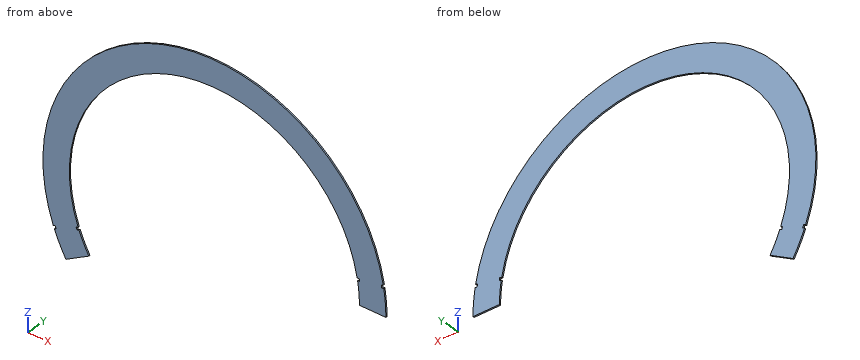
from build123d import *

# Parameters (mm, degrees)
BOSS_EXTRUDE1_DEPTH = 0.7
CUT_EXTRUDE1_DEPTH  = 120.107123213
BOSS_EXTRUDE2_DEPTH = 0.7


with BuildPart() as part:
    # Sketch3 → Boss-Extrude1 (new body)
    with BuildSketch(Plane(origin=(0, 0, 0), x_dir=(1, 0, 0), z_dir=(0, 1, 0))):
        with BuildLine():
            Line((-61.678329258, 35.61), (-72.936659507, 42.11))
            ThreePointArc((-72.936659507, 42.11), (-21.797739979, -81.35027309), (84.22, 0))
            Line((84.22, 0), (71.22, 0))
            ThreePointArc((71.22, 0), (-18.433092392, -68.793237348), (-61.678329258, 35.61))
        make_face()
    extrude(amount=BOSS_EXTRUDE1_DEPTH)

    # Sketch5 → Cut-Extrude1 (cut, through all)
    with BuildSketch(Plane(origin=(0, 0, 0), x_dir=(1, 0, 0), z_dir=(0, 1, 0))):
        Polygon((-66.489597975, 25.522965367), (-80.493304373, 30.89848461), (-81.020297764, 29.488976758), (-66.924908452, 24.358674608), align=None)
    cut_extrude1 = extrude(amount=CUT_EXTRUDE1_DEPTH, mode=Mode.SUBTRACT)


with BuildPart() as cut_extrude1_piece_1:
    # of the separate pieces the step leaves, piece 1, a body of its own (cut_extrude1_pieces)
    add(part.part.solids().sort_by_distance((84.22, 0, 0))[0])



with BuildPart() as cut_extrude1_piece_2:
    # of the separate pieces the step leaves, piece 2, a body of its own (cut_extrude1_pieces)
    add(part.part.solids().sort_by_distance((-72.936659507, 0, -42.11))[0])


with BuildPart() as cut_extrude1_piece_1_1:
    add(cut_extrude1_piece_1.part)

    add(cut_extrude1_piece_2.part)  # Boss-Extrude2 merges Cut-Extrude1 piece 2
    # Sketch6 → Boss-Extrude2 (add)
    with BuildSketch(Plane(origin=(0, 0, 0), x_dir=(1, 0, 0), z_dir=(0, 1, 0))):
        Polygon((-77.692563093, 29.823380761), (-67.423178402, 25.881333316), (-67.943747449, 24.525204583), (-78.213132141, 28.467252028), align=None)
    boss_extrude2 = extrude(amount=BOSS_EXTRUDE2_DEPTH)

    # Mirror1: Cut-Extrude1, Boss-Extrude2 across plane
    add(cut_extrude1.mirror(Plane(origin=(0, 0, 0), x_dir=(-0.25881904510251774, 0, 0.9659258262890691), z_dir=(0.9659258262890692, 0, 0.25881904510251774))), mode=Mode.SUBTRACT)
    add(boss_extrude2.mirror(Plane(origin=(0, 0, 0), x_dir=(-0.25881904510251774, 0, 0.9659258262890691), z_dir=(0.9659258262890692, 0, 0.25881904510251774))))


solid = cut_extrude1_piece_1_1.part
Check sheet for the modelled part. Datum: model origin and axes. Units: mm. Round coordinates to 2 decimals unless told otherwise and drop trailing zeros. Order: outer loops, then holes, each group sorted by start corner. A loop starts at its lowest first (then second) coordinate and runs counter-clockwise, first axis right, second up. Notation, with made-up numbers: M 44.25,-7.75 L 84.25,-7.75 A20 ccw 84.25,11.25 Z; hole C -2.5,59.25 d4. An arc over 180 degrees is marked long. One line per item, written item: value. Start each with the question number.
1. Section check C-C on x = 0. Enter the section's corners in (y, z).
2. Section check D-D on z = 38.5. Enter the section's corners in (x, y) (3 decimals).
3. Gauge pin test, flat end, axial feed: P1, Ø12, axis at x = 55, z = 67, coming from the +Y side. Record the tip position at first contact, or that the pin passes through.
4. Scan lines: line 1 along Z through (x, y) = (0, 0.65); line 2 along X through (y, z) = (0.25, 62); line 3 along X through (y, z) = (0.1, 19). Record each from-to range of solid material in increasing order.
5. Section check B-B on y = 0.3. Enter the section's corners in (x, z), and give its area (3 significant figures).
6. Section check A-A on z = 53.5. Enter the section's corners in (x, y).
Results found:
1. outline: M 0,71.22 L 0.7,71.22 L 0.7,84.22 L 0,84.22 Z
2. outline: M -74.905,0 L -59.917,0 L -59.917,0.7 L -74.905,0.7 Z; M 59.917,0 L 74.905,0 L 74.905,0.7 L 59.917,0.7 Z
3. P1: y = 0.7
4. line 1: 71.22 to 84.22
4. line 2: -57 to -35.05, 35.05 to 57
4. line 3: -82.05 to -68.64, 68.64 to 82.05
5. outline: M -79.14,-28.8 L -78.21,-28.47 L -77.69,-29.82 L -78.63,-30.18 A84.22 ccw -72.94,-42.11 L -61.68,-35.61 A71.22 cw -66.49,-25.52 L -67.42,-25.88 L -67.87,-24.7 L -66.92,-24.36 A71.22 cw long 70.14,12.37 L 71.13,12.54 L 71.33,11.3 L 70.34,11.14 A71.22 cw 71.22,0 L 84.22,0 A84.22 ccw 83.18,13.17 L 82.2,13.02 L 81.97,14.45 L 82.94,14.62 A84.22 ccw long Z
5. area: 3,700 mm^2
6. outline: M -65.04,0 L -47.01,0 L -47.01,0.7 L -65.04,0.7 Z; M 47.01,0 L 65.04,0 L 65.04,0.7 L 47.01,0.7 Z
